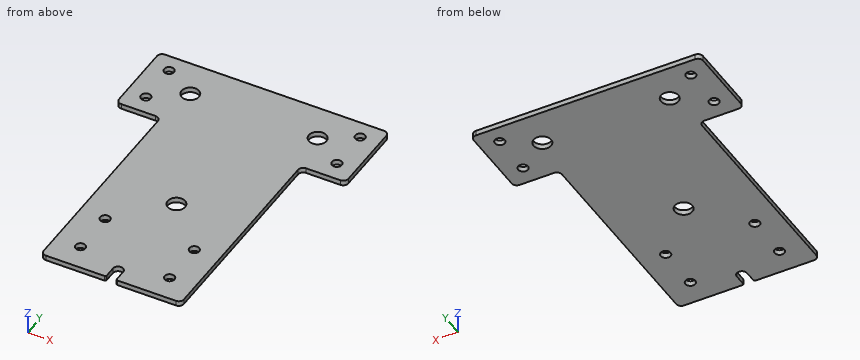
from build123d import *

# Parameters (mm, degrees)
SKETCH1_W                                 = 2.58826
SKETCH1_H                                 = 152.4
BASE_FLANGE1_DEPTH                        = 69.85
SKETCH2_W                                 = 22.225
SKETCH2_H                                 = 44.45
BOSS_EXTRUDE1_DEPTH                       = 2.58826
F_10_0_1935_DIAMETER_HOLE1_D              = 4.9149
SKETCH5_W                                 = 114.3
SKETCH5_H                                 = 5.16255
CUT_EXTRUDE1_DEPTH                        = 179.073762006
FILLET1_R                                 = 2.54
HOLE_FOR_1_4_SELF_CLINCHING_NUTS_S_SS_C_D = 8.7376
CUT_EXTRUDE2_DEPTH                        = 179.073762006
FILLET2_R                                 = 0.762


# Sheet-metal steps are written as plain solids
with BuildPart() as part:
    # Sketch1 → Base-Flange1 (new body)
    with BuildSketch(Plane(origin=(0, 0, 0), x_dir=(0, 0, -1), z_dir=(1, 0, 0))):
        with Locations((-1.29413, -76.2)):
            Rectangle(SKETCH1_W, SKETCH1_H)
    extrude(amount=BASE_FLANGE1_DEPTH)

    # Sketch2 → Boss-Extrude1 (add)
    with BuildSketch(Plane(origin=(0, 0, 0), x_dir=(-1, 0, 0), z_dir=(0, 0, -1))):
        with Locations((-80.9625, -22.225)):
            Rectangle(SKETCH2_W, SKETCH2_H)
        with Locations((11.1125, -22.225)):
            Rectangle(SKETCH2_W, SKETCH2_H)
    extrude(amount=-BOSS_EXTRUDE1_DEPTH)

    # #10 (0.1935) Diameter Hole1 (through all)
    with Locations(Plane(origin=(0, 0, 0), x_dir=(-1, 0, 0), z_dir=(0, 0, -1))):
        with Locations((-82.55, -13.97), (-82.55, -34.925), (12.7, -34.925), (12.7, -13.97), (-57.15, -117.475), (-57.15, -139.7), (-12.7, -139.7), (-12.7, -117.475)):
            Hole(F_10_0_1935_DIAMETER_HOLE1_D / 2)

    # Sketch5 → Cut-Extrude1 (cut, through all)
    with BuildSketch(Plane(origin=(0, 0, 0), x_dir=(-1, 0, 0), z_dir=(0, 0, -1))):
        with Locations((-34.925, -2.581275)):
            Rectangle(SKETCH5_W, SKETCH5_H)
    extrude(amount=-CUT_EXTRUDE1_DEPTH, mode=Mode.SUBTRACT)

    # Fillet1
    fillet1_edges = [part.edges().sort_by_distance(p)[0] for p in [
        (92.075, -44.45, 1.29413),
        (69.85, -44.45, 1.29413),
        (69.85, -152.4, 1.29413),
        (0, -44.45, 1.29413),
        (-22.225, -44.45, 1.29413),
        (0, -152.4, 1.29413),
        (92.075, -5.16255, 1.29413),
        (-22.225, -5.16255, 1.29413),
    ]]
    fillet(fillet1_edges, radius=FILLET1_R)

    # Hole for 1/4 Self-clinching Nuts (S,SS,CLS,CLSS)1 (through all)
    with Locations(Plane(origin=(0, 0, 0), x_dir=(-1, 0, 0), z_dir=(0, 0, -1))):
        with Locations((-66.675, -23.622), (-3.175, -23.622), (-34.925, -93.472)):
            Hole(HOLE_FOR_1_4_SELF_CLINCHING_NUTS_S_SS_C_D / 2)

    # Sketch8 → Cut-Extrude2 (cut, through all)
    with BuildSketch(Plane(origin=(0, 0, 0), x_dir=(-1, 0, 0), z_dir=(0, 0, -1))):
        with BuildLine():
            Line((-37.465, -152.4), (-37.465, -146.05))
            ThreePointArc((-37.465, -146.05), (-34.925, -143.51), (-32.385, -146.05))
            Line((-32.385, -146.05), (-32.385, -152.4))
            Line((-32.385, -152.4), (-37.465, -152.4))
        make_face()
    extrude(amount=-CUT_EXTRUDE2_DEPTH, mode=Mode.SUBTRACT)

    # Fillet2
    fillet2_edges = [part.edges().sort_by_distance(p)[0] for p in [
        (32.385, -152.4, 1.29413),
        (37.465, -152.4, 1.29413),
    ]]
    fillet(fillet2_edges, radius=FILLET2_R)


solid = part.part
Can you work these out from the model? Positions are in its coordinate system, mm. Coordinates: 2 decimals unless noted, no trailing zeros. Loops run counter-clockwise (first coordinate to the right, second up) from the corner with the lowest first, then second, coordinate; pieces in that order, holes last. Notation, with made-up numbers: M 4,80 L 21,80 A24 cw 21,106 Z; hole C 45,79 d7. An arc over 180 degrees is marked long. Return JSON: item names as keys, results as strings. Group by question number.
Item 1: Imagine slicing it at A-A (y = -139.7). Please give me the cut outline in (x, z).
Item 2: Imagine slicing it at D-D (z = 1.7). Give the number of separate pieces and of enclosed holes in the cut face, and give its area (3 significant figures).
Item 3: Imagine slicing it at B-B (x = 82.55). Please give me the cut outline in (y, z), and give its area (3 significant figures).
Item 4: Imagine slicing it at C-C (y = -95). Please give me the cut outline in (x, z), and give its area (3 significant figures).
Item 5: If I drill on L1, parallel to Y at x = 82.55, z = 0.6; L2, parallel to X at y = -139.7, z = 1.85; L3, parallel to Y at x = 57.15, z = 0.65, over which ranges is the centre line in solid material (lowest first)? Write a range as from..to.
Item 6: I'm going to push flat-ended pins straight in: pin 1 Ø1.5 at (y, z) = (-68, 0.5) entering from +X; pin 2 Ø0.8 at (y, z) = (-148.5, 0.5) entering from -X. Where does each tip first touch, or does it pass through?
Verdict:
{
 "1": {"outline": "M 0,0 L 10.24,0 L 10.24,2.59 L 0,2.59 Z; M 15.16,0 L 54.69,0 L 54.69,2.59 L 15.16,2.59 Z; M 59.61,0 L 69.85,0 L 69.85,2.59 L 59.61,2.59 Z"},
 "2": {"separate pieces": "1", "enclosed holes": "11", "area": "11,700 mm^2"},
 "3": {"outline": "M -44.45,0 L -37.38,0 L -37.38,2.59 L -44.45,2.59 Z; M -32.47,0 L -16.43,0 L -16.43,2.59 L -32.47,2.59 Z; M -11.51,0 L -5.16,0 L -5.16,2.59 L -11.51,2.59 Z", "area": "76.2 mm^2"},
 "4": {"outline": "M 0,0 L 30.83,0 L 30.83,2.59 L 0,2.59 Z; M 39.02,0 L 69.85,0 L 69.85,2.59 L 39.02,2.59 Z", "area": "160 mm^2"},
 "5": {"L1": "y = -44.45..-37.38, -32.47..-16.43, -11.51..-5.16", "L2": "x = 0..10.24, 15.16..54.69, 59.61..69.85", "L3": "y = -152.4..-142.16, -137.24..-119.93, -115.02..-5.16"},
 "6": {"pin 1": "stops at x = 69.85", "pin 2": "stops at x = 0"}
}
